```python
from build123d import *

# Parameters (mm, degrees)
F0_W     = 150
F0_H     = 50
F1_DEPTH = 50
F2_DEPTH = 25
F0_W_2   = 25


with BuildPart() as f1:
    # F0 (on Front) → F1 (new body, symmetric)
    with BuildSketch(Plane.XZ):
        with Locations((-75, -25)):
            Rectangle(F0_W, F0_H)
    extrude(amount=F1_DEPTH, both=True)

    # F0 (on Front) → F2 (join, symmetric)
    with BuildSketch(Plane.XZ):
        with BuildLine():
            Line((-150, 0), (0, 0))
            ThreePointArc((0, 0), (14.644661, 35.355339), (50, 50))
            Line((50, 50), (50, 100))
            add(Edge.make_bspline(
                [(-150, 0), (-146.281272, 63.885584), (-17.262463, 65.02264), (50, 100)],
                knots=[0, 0, 0, 0, 223.606798, 223.606798, 223.606798, 223.606798], degree=3))
        make_face()
    extrude(amount=F2_DEPTH, both=True)

    # F0 (on Front) → F3 (revolve)
    with BuildSketch(Plane.XZ):
        with Locations((62.5, 75)):
            Rectangle(F0_W_2, F0_H)
    revolve(axis=Axis((50, 0, 75), (0, 0, 1)))


solid = f1.part
```
For this review, take the finished solid that the model builds, in its own axes (mm). A direction names the side the tool comes from. Round coordinates to 2 decimals unless told otherwise and drop trailing zeros. Loops run counter-clockwise (first coordinate to the right, second up) from the corner with the lowest first, then second, coordinate; pieces in that order, holes last.
(1) We need section A-A (z = -23.5). Give the boundary of the cut face in (x, y).
Returned:
outline: (-150, -50) - (0, -50) - (0, 50) - (-150, 50) - close
(2) Clearance check with flat-ended pins moving along their axes: P1, Ø5, axis at y = -5.5, z = 4.5, coming from the +X side; P2, Ø1.5, axis at x = -46, z = 61.5, coming from the +Y side; P3, Ø7.5, axis at x = 63, y = -6.5, coming from the -Z side. State where each tip first meets the part, or that it passes through.
Returned:
P1: stops at x = 0.49
P2: stops at y = 25
P3: stops at z = 50
(3) We need section B-B (y = -28.5). Give the boundary of the cut face in (x, z), plus the area to 3 significant figures.
Returned:
outline: (-150, -50) - (0, -50) - (0, 0) - (-150, 0) - close
area: 7,500 mm2
(4) Wall thickness on line 1 along Z through (x, y) = (-139.5, 40.5); line 2 along X through (y, z) = (-30.5, -5); line 3 along Y through (x, z) = (-92.5, 20.5): over which ranges is each line inside the solid? List them lowest first.
Returned:
line 1: z = -50 to 0
line 2: x = -150 to 0
line 3: y = -25 to 25
(5) Tool access review of faces 1 (the flat face through (-76, -1, -50)), 2 (the cylindrical face through (25.006, 0.55, 95.9)), 3 (the flat face through (-76, -38, 0)), 4 (the flat face through (-51, 25, 40)), 5 (the flat face through (60, 0, 50)): name each direction out of +Z, -Z, +X, -X, +Y, -Y from which nothing blocks a thin tool from reaching the whole face with its end or side.
Returned:
face 1: -Z, +X, -X, +Y, -Y
face 2: +Z, -X
face 3: +Z, +X, -X, -Y
face 4: +Z, +X, -X, +Y
face 5: -Z, +X, +Y, -Y
